The listing builds one solid part. Answer for the finished solid, in the listing's coordinates (mm). Face numbers are marked on the shaded views. Give positions to 0.01 mm unless a question says otherwise; leave off trailing zeros. Order: outer loops, then holes, each group sorted by start corner. A loop starts at its lowest first (then second) coordinate and runs counter-clockwise, first axis right, second up. Notation, with made-up numbers: (-32, -28.5) - (-18, -28.5) arc R6 cw to (-18, -19.5) - close; hole circle Ø8 at (75, 35). An arc over 180 degrees is marked (long way). Answer in a Markdown table with one row per item.
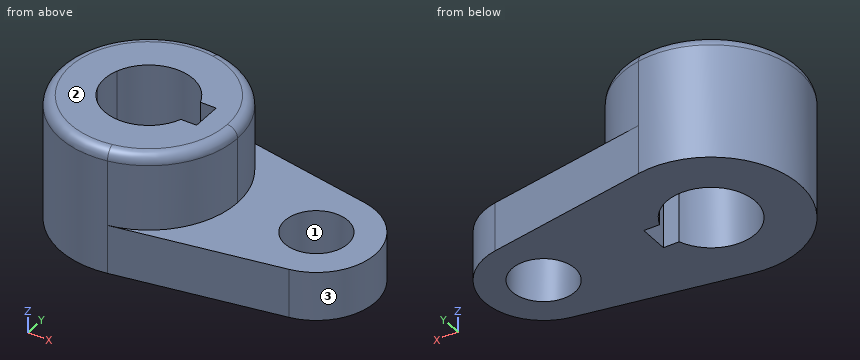
from build123d import *

# Parameters (mm, degrees)
F1_DEPTH = 40.2336
F0_R     = 10.16
F2_DEPTH = 15.7734
F3_R     = 3.302


with BuildPart() as f1:
    # F0 (on Top) → F1 (new body)
    with BuildSketch(Plane.XY):
        with BuildLine():
            ThreePointArc((-30.901911, -28.126541), (-14.028534, -18.336262), (-7.369558, 0))
            ThreePointArc((-7.369558, 0), (-14.028534, 18.336262), (-30.901911, 28.126541))
            ThreePointArc((-30.901911, 28.126541), (-64.519558, 0), (-30.901911, -28.126541))
        make_face()
        with BuildLine():
            ThreePointArc((-49.392323, -4.826), (-50.232058, 0), (-49.392323, 4.826))
            ThreePointArc((-49.392323, 4.826), (-35.944558, 14.2875), (-22.496793, 4.826))
            Line((-22.496793, 4.826), (-17.415258, 4.826))
            Line((-17.415258, 4.826), (-17.415258, -4.826))
            Line((-17.415258, -4.826), (-22.496793, -4.826))
            ThreePointArc((-22.496793, -4.826), (-35.944558, -14.2875), (-49.392323, -4.826))
        make_face(mode=Mode.SUBTRACT)
    extrude(amount=F1_DEPTH)

    # F0 (on Top) → F2 (join)
    with BuildSketch(Plane.XY):
        with BuildLine():
            ThreePointArc((-30.901911, 28.126541), (-14.028534, 18.336262), (-7.369558, 0))
            ThreePointArc((-7.369558, 0), (-14.028534, -18.336262), (-30.901911, -28.126541))
            Line((-30.901911, -28.126541), (21.392206, -18.751028))
            ThreePointArc((21.392206, -18.751028), (37.080442, 0), (21.392206, 18.751028))
            Line((21.392206, 18.751028), (-30.901911, 28.126541))
        make_face()
        with Locations((18.030442, 0)):
            Circle(F0_R, mode=Mode.SUBTRACT)
    extrude(amount=F2_DEPTH)

    # F3
    f3_edges = [f1.edges().sort_by_distance(p)[0] for p in [
        (-40.987205, 28.126541, 40.2336),
    ]]
    fillet(f3_edges, radius=F3_R)


solid = f1.part
Item 1: Determine the mould class of the marked faces 1, 2 and 3 for opening direction Y: pulls with the +Y half, pulls with the -Y half, needs draft (parallel to the pull), parting line crosses it, or undercut.
Answer block:
| item | result |
|---|---|
| face 1 | undercut |
| face 2 | needs draft |
| face 3 | parting line crosses it |
Item 2: Consider line 1 (Z direction, x = 1.5, y = 1); line 2 (X direction, y = 4, z = 14.5); line 3 (X direction, y = -9, z = 15.5). Determine where each line is inside the solid, lowest interval first.
Answer block:
| item | result |
|---|---|
| line 1 | 0 to 15.77 |
| line 2 | -64.24 to -49.66, -17.42 to 8.69, 27.37 to 36.66 |
| line 3 | -63.07 to -47.04, -24.85 to 13.32, 22.74 to 34.82 |
Item 3: Each of these flat-tipped pins is pushed along its axis until it touches: P1, Ø12, axis at x = 18.03, y = 0, coming from the -Z side; P2, Ø2, axis at y = 7, z = 4, coming from the -X side; P3, Ø2, axis at y = -17.5, z = 34, coming from the +X side; P4, Ø1.5, axis at y = -3.5, z = 7, coming from the -X side. Where does it stop, or does it pass through?
Answer block:
| item | result |
|---|---|
| P1 | through |
| P2 | x = -63.88 |
| P3 | x = -12.61 |
| P4 | x = -64.39 |
Item 4: Find section D-D on x = 3. Write down the section's boundary in (y, z), then the cut area to 3 significant figures.
Answer block:
| item | result |
|---|---|
| outline | (-22.05, 0) - (22.05, 0) - (22.05, 15.77) - (-22.05, 15.77) - close |
| area | 696 mm² |
Item 5: Find section A-A on z = 10. Count the separate pieces of the cut face and the enclosed holes in it, then the cut area to 3 significant figures.
Answer block:
| item | result |
|---|---|
| separate pieces | 1 |
| enclosed holes | 2 |
| area | 3,450 mm² |
